```python
from build123d import *

# Parameters (mm, degrees)
F1_DEPTH = 4
F2_R     = 4
F5_W     = 1
F5_H     = 1.5


with BuildPart() as f1:
    # F0 (on Top) → F1 (new body)
    with BuildSketch(Plane.XY):
        with BuildLine():
            Line((0, 8), (0, 0))
            Line((0, 0), (16, 0))
            Line((16, 0), (16, 8))
            Line((16, 8), (14, 8))
            ThreePointArc((14, 8), (8, 2), (2, 8))
            Line((2, 8), (0, 8))
        make_face()
    extrude(amount=F1_DEPTH)

    # F2
    f2_edges = [f1.edges().sort_by_distance(p)[0] for p in [
        (16, 0, 2),
        (0, 0, 2),
    ]]
    fillet(f2_edges, radius=F2_R)

    # F6: sweep along a path in F4
    with BuildLine(Plane.XY.offset(2)) as f6_path:
        ThreePointArc((1, 8), (8, 1), (15, 8))
    # F5 (on face) → F6 (sweep, cut)
    with BuildSketch(Plane(origin=(0, 8, 0), x_dir=(-1, 0, 0), z_dir=(0, 1, 0))):
        with Locations((-1, 2)):
            Rectangle(F5_W, F5_H)
    sweep(path=f6_path.line, mode=Mode.SUBTRACT)


solid = f1.part
```
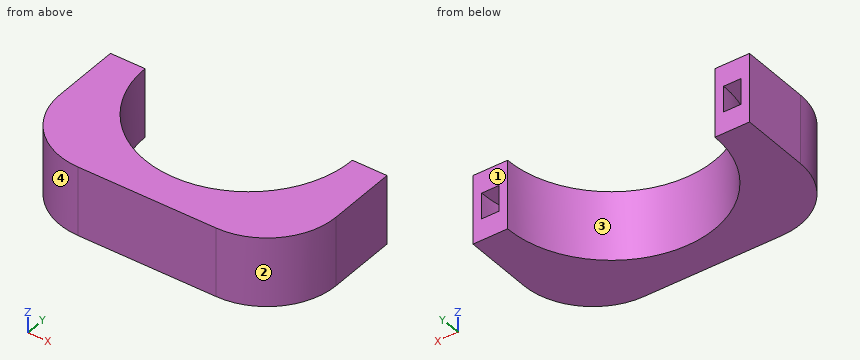
The listing builds one solid part. Answer for the finished solid, in the listing's coordinates (mm). Face numbers are marked on the shaded views. Coordinates: 2 decimals unless noted, no trailing zeros. Write each loop counter-clockwise with the first axis right and the second up, starting at its lowest first coordinate (ties: lowest second). Pieces come first, ordered by that corner, then holes. Notation, with made-up numbers: (5, 24.25) - (42, 24.25) arc R14 cw to (42, 46.25) - close; hole circle Ø5 at (35, -19). An arc over 180 degrees is marked (long way). Return JSON: item names as keys, results as strings. Group by question number.
Q1. The part is cut by section A-A on z = 1.95. Write down the section's boundary in (x, y), and give its area (3 significant figures).
Q2. Find the intervals of material crossed by line 1 along Z through (x, y) = (1, 7); line 2 along X through (y, z) = (4.5, 1.7); line 3 along X through (y, z) = (2.5, 0.55), in increasing order. Write a range as [from, to].
Q3. The part is cut by section D-D on z = 0.7. Write down the section's boundary in (x, y).
Q4. A flat-ended cylindrical pin translates along its axis: pin 1 Ø1.5 at (y, z) = (2.5, 2) entering from +X. Find the tip coordinate at first contact, or state that the pin passes through.
Q5. The part is cut by section B-B on y = 5.5. Write down the section's boundary in (x, z).
Q6. For a pull along X with two mould halves and no side action, classify the marked faces 1, 2, 3 and 4 as +X half, -X half, draft (parallel to the pull), parting line (faces both ways), or undercut.
Q7. The part is cut by section C-C on x = 8. Write down the section's boundary in (y, z), and give its area (3 significant figures).
Evaluation:
{
 "1": {"outline": "(0, 4) arc R4 ccw to (4, 0) - (12, 0) arc R4 ccw to (16, 4) - (16, 8) - (15.5, 8) arc R7.5 cw to (0.5, 8) - (0, 8) - close; (1.5, 8) arc R6.5 ccw to (14.5, 8) - (14, 8) arc R6 cw to (2, 8) - close", "area": "42.6 mm2"},
 "2": {"line 1": "z = [0, 1.25], [2.75, 4]", "line 2": "x = [0, 1.37], [2.52, 3.13], [12.87, 13.48], [14.63, 16]", "line 3": "x = [0.29, 5.6], [10.4, 15.71]"},
 "3": {"outline": "(0, 4) arc R4 ccw to (4, 0) - (12, 0) arc R4 ccw to (16, 4) - (16, 8) - (14, 8) arc R6 cw to (2, 8) - (0, 8) - close"},
 "4": {"pin 1": "stops at x = 15.93"},
 "5": {"outline": "(0, 0) - (2.55, 0) - (2.55, 4) - (0, 4) - close; (13.45, 0) - (16, 0) - (16, 4) - (13.45, 4) - close; hole (0.93, 1.25) - (2, 1.25) - (2, 2.75) - (0.93, 2.75) - close; hole (14, 1.25) - (15.07, 1.25) - (15.07, 2.75) - (14, 2.75) - close"},
 "6": {"face 1": "draft", "face 2": "+X half", "face 3": "undercut", "face 4": "-X half"},
 "7": {"outline": "(0, 0) - (2, 0) - (2, 4) - (0, 4) - close; hole (0.5, 1.25) - (1.5, 1.25) - (1.5, 2.75) - (0.5, 2.75) - close", "area": "6.50 mm2"}
}
